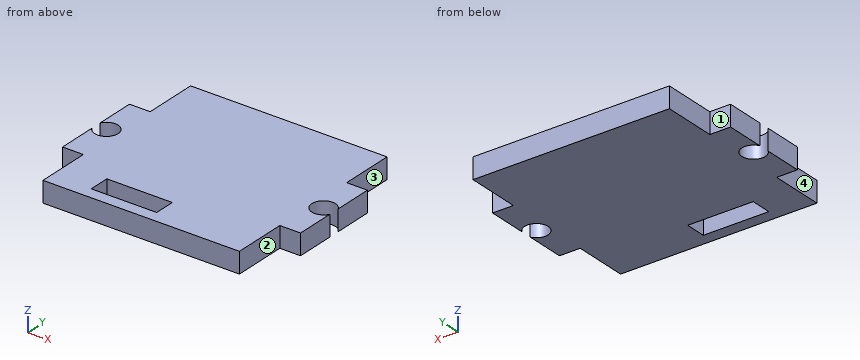
```python
from build123d import *

# Parameters (mm, degrees)
SKETCH1_W           = 10
SKETCH1_H           = 3.175
BOSS_EXTRUDE4_DEPTH = 3.175


with BuildPart() as part:
    # Sketch1 → Boss-Extrude4 (new body)
    with BuildSketch(Plane.XY):
        with BuildLine():
            Line((-33.68050161, 39.580766243), (-36.85550161, 39.580766243))
            Line((-36.85550161, 39.580766243), (-36.85550161, 33.629202304))
            ThreePointArc((-36.85550161, 33.629202304), (-33.46800161, 32.780766243), (-36.85550161, 31.932330182))
            Line((-36.85550161, 31.932330182), (-36.85550161, 25.980766243))
            Line((-36.85550161, 25.980766243), (-33.68050161, 25.980766243))
            Line((-33.68050161, 25.980766243), (-33.68050161, 17.780766243))
            Line((-33.68050161, 17.780766243), (-3.68050161, 17.780766243))
            Line((-3.68050161, 17.780766243), (-3.68050161, 25.980766243))
            Line((-3.68050161, 25.980766243), (-0.50550161, 25.980766243))
            Line((-0.50550161, 25.980766243), (-0.50550161, 31.932330182))
            ThreePointArc((-0.50550161, 31.932330182), (-3.89300161, 32.780766243), (-0.50550161, 33.629202304))
            Line((-0.50550161, 33.629202304), (-0.50550161, 39.580766243))
            Line((-0.50550161, 39.580766243), (-3.68050161, 39.580766243))
            Line((-3.68050161, 39.580766243), (-3.68050161, 47.780766243))
            Line((-3.68050161, 47.780766243), (-33.68050161, 47.780766243))
            Line((-33.68050161, 47.780766243), (-33.68050161, 39.580766243))
        make_face()
        with Locations((-22.68050161, 21.182701237)):
            Rectangle(SKETCH1_W, SKETCH1_H, mode=Mode.SUBTRACT)
    extrude(amount=BOSS_EXTRUDE4_DEPTH)


solid = part.part
```
Geometry: final body of the model. Coordinates: model frame, mm. Face numbers are marked on the shaded views. A direction names the side the tool comes from. Give positions to 0.01 mm unless a question says otherwise; leave off trailing zeros. Order: outer loops, then holes, each group sorted by start corner. A loop starts at its lowest first (then second) coordinate and runs counter-clockwise, first axis right, second up. Notation, with made-up numbers: M -13.75,59 L 23.25,59 A31 cw 23.25,86 Z; hole C 66.5,3 d6. An arc over 180 degrees is marked long. Answer as CSV lines item,"result". Start each with the question number.
1) Cut plane B-B (y = 22). Output: boundary loops of the cut face in (x, z) (1 decimal).
2) Set-up query: the marked faces 1, 2, 3 and 4. Return all of +Z, -Z, +X, -X, +Y, -Y with unobstructed straight access to the full face (end or side cutting, diameter ignored); none if empty.
3) Cut plane C-C (z = 2.5). Output: boundary loops of the cut face in (x, y), then the cut area to 3 significant figures.
4) Cut plane A-A (x = -24.5). Output: boundary loops of the cut face in (y, z) (3 decimals).
5) First-contact query: P1, Ø1.6, axis at y = 41.5, z = 1, coming from the +X side; P2, Ø3, axis at x = -35.27, y = 32.78, coming from the -Z side; P3, Ø1, axis at x = -3, z = 2.5, coming from the +Y side. Flat tips, straight axial feed; report the tip coordinate or a pass-through.
6) Cut plane D-D (y = 44.5). Output: boundary loops of the cut face in (x, z) (1 decimal), then the cut area to 4 significant figures.
7) Line query: line 1 (Y direction, x = -20.5, z = 2.25); line 2 (Y direction, x = -2, z = 0.25); line 3 (X direction, y = 22.5, z = 2.4). Output: solid intervals per line, ascending. Write a range as from..to.
Findings below:
1,outline,"M -33.7,0 L -27.7,0 L -27.7,3.2 L -33.7,3.2 Z; M -17.7,0 L -3.7,0 L -3.7,3.2 L -17.7,3.2 Z"
2,face 1,"+Z, -Z, -X, +Y"
2,face 2,"+Z, -Z, +X, -Y"
2,face 3,"+Z, -Z, +X, +Y"
2,face 4,"+Z, -Z, -X, -Y"
3,outline,"M -36.86,25.98 L -33.68,25.98 L -33.68,17.78 L -3.68,17.78 L -3.68,25.98 L -0.51,25.98 L -0.51,31.93 A1.8 cw long -0.51,33.63 L -0.51,39.58 L -3.68,39.58 L -3.68,47.78 L -33.68,47.78 L -33.68,39.58 L -36.86,39.58 L -36.86,33.63 A1.8 cw long -36.86,31.93 Z; hole M -27.68,19.6 L -17.68,19.6 L -17.68,22.77 L -27.68,22.77 Z"
3,area,"935 mm²"
4,outline,"M 17.781,0 L 19.595,0 L 19.595,3.175 L 17.781,3.175 Z; M 22.77,0 L 47.781,0 L 47.781,3.175 L 22.77,3.175 Z"
5,P1,"stops at x = -3.68"
5,P2,"passes through"
5,P3,"stops at y = 39.58"
6,outline,"M -33.7,0 L -3.7,0 L -3.7,3.2 L -33.7,3.2 Z"
6,area,"95.25 mm²"
7,line 1,"y = 17.78..19.6, 22.77..47.78"
7,line 2,"y = 25.98..30.98, 34.58..39.58"
7,line 3,"x = -33.68..-27.68, -17.68..-3.68"
